Check sheet for the modelled part. Datum: model origin and axes. Units: mm. A direction names the side the tool comes from. Give positions to 0.01 mm unless a question says otherwise; leave off trailing zeros. Write each loop counter-clockwise with the first axis right and the second up, starting at its lowest first coordinate (ties: lowest second). Pieces come first, ordered by that corner, then holes. Notation, with made-up numbers: (15, 47) -> (41, 47) arc R26 cw to (41, 78) -> close; hole circle Ø9 at (36.25, 55). An arc over 180 degrees is marked (long way). Answer as a JSON object with one key per item and string values.
Autodesk Inventor part; units mm, degrees
ref_plane "Work Plane2" through (-40.9959, 0.8639, 22.2359) normal (0, 0, 1) x (1, 0, 0)
ref_plane "YZ Plane" through (0, 0, 0) normal (1, 0, 0) x (0, 1, 0)
ref_plane "XZ Plane" through (0, 0, 0) normal (0, 1, 0) x (-1, 0, 0)
ref_plane "Work Plane1" through (0, 0, 10) normal (0, 0, 1) x (1, 0, 0)
sketch "Sketch1" plane through (0, 0, 10) normal (0, 0, 1) x (1, 0, 0)
  line L0 (-4.0299, -0.3538) -> (-2.2322, 1.4439) construction
  arc A0 (-1.4439, 2.2322) -> (-2.2322, 1.4439) centre (-0.9299, 0.9299) ccw construction
  line L1 (-1.4439, 2.2322) -> (0.3538, 4.0299) construction
  line L2 (-37.8299, 42.8299) -> (-37.8299, 37.8299) construction
  line L3 (-37.8299, 37.8299) -> (-42.9208, 37.8299) construction
  line L4 (-37.8299, 42.2137) -> (-37.8299, 45.8299) construction
  line L5 (-37.8299, 45.8299) -> (-4.0299, 45.8299) construction
  line L6 (-4.0299, 45.8299) -> (-4.0299, 42.2137) construction
  line L7 (-4.0299, 4.0299) -> (0.3538, 4.0299)
  circle A1 centre (-20.9299, 20.9299) radius 17.5
  line L8 (-20.9299, 58.9723) -> (17.1124, 20.9299) construction
  line L9 (17.1124, 20.9299) -> (-20.9299, -17.1124) construction
  line L10 (-20.9299, -17.1124) -> (-58.9723, 20.9299) construction
  line L11 (-58.9723, 20.9299) -> (-20.9299, 58.9723) construction
  line L12 (-20.9299, 58.9723) -> (-20.9299, -17.1124) construction
  line L13 (17.1124, 20.9299) -> (-58.9723, 20.9299) construction
  line L14 (-20.9299, 58.9723) -> (32.8701, 58.9723) construction
  line L15 (-43.4299, 43.4299) -> (1.5701, 43.4299) construction
  line L16 (1.5701, 43.4299) -> (1.5701, -1.5701) construction
  line L17 (1.5701, -1.5701) -> (-43.4299, -1.5701) construction
  line L18 (-43.4299, -1.5701) -> (-43.4299, 43.4299) construction
  line L19 (-43.4299, 43.4299) -> (1.5701, -1.5701) construction
  line L20 (1.5701, 43.4299) -> (-43.4299, -1.5701) construction
  line L21 (-43.4299, 5.3876) -> (-43.4299, 36.4723)
  line L22 (-43.4299, 36.4723) -> (-36.4723, 43.4299)
  line L23 (-36.4723, 43.4299) -> (-5.3876, 43.4299)
  line L24 (-5.3876, 43.4299) -> (1.5701, 36.4723)
  line L25 (1.5701, 36.4723) -> (1.5701, 5.3876)
  line L26 (1.5701, 5.3876) -> (-5.3876, -1.5701)
  line L27 (-5.3876, -1.5701) -> (-36.4723, -1.5701)
  line L28 (-36.4723, -1.5701) -> (-43.4299, 5.3876)
  line L29 (-4.0299, 42.2137) -> (-37.8299, 42.2137)
  line L30 (-4.0299, -0.3538) -> (-4.0299, 4.0299)
  point P0 (-37.8299, 4.0299)
  point P1 (-20.9299, 20.9299)
  dimension "d18" = 53.8
  dimension "d19" = 45
  dimension "d20" = 53.8
  dimension "d21" = 45
  dimension "d22" = 45
extrude "Extrusion1" add sketch "Sketch1" along normal blind 5
sketch "Sketch2" plane through (0, 0, 15) normal (0, 0, 1) x (1, 0, 0)
  circle A0 centre (-35.9299, 35.9299) radius 3.0099 construction
  circle A1 centre (-5.93, 35.9299) radius 3.0099 construction
  circle A2 centre (-5.93, 5.93) radius 3.0099 construction
  circle A3 centre (-35.9299, 5.93) radius 3.0099 construction
  circle A4 centre (-35.9299, 35.9299) radius 2.7099
  circle A5 centre (-5.93, 35.9299) radius 2.7099
  circle A6 centre (-5.93, 5.93) radius 2.7099
  circle A7 centre (-35.9299, 5.93) radius 2.7099
  point P0 (0, 0)
  dimension "d_1" = 0.3
  dimension "d13" = 0.3
  dimension "d14" = 0.3
  dimension "d15" = 0.3
ref_plane "Work Plane2" through (-40.9959, 0.8639, 22.2359) normal (0, 0, 1) x (1, 0, 0)
extrude "Extrusion2" add sketch "Sketch2" along normal up to surface (7.2359 mm away)
sketch "Sketch3" plane through (0, 0, 10) normal (0, 0, -1) x (-1, 0, 0)
  line L0 (37.8299, -0.4701) -> (37.8299, 4.0299) construction
  line L1 (4.0299, 4.0299) -> (4.0299, -0.4701) construction
  line L2 (37.8299, -0.4701) -> (37.8299, 1.1886) construction
  line L3 (4.0299, -3.9701) -> (4.0299, -0.3538) construction
  line L4 (45.8299, 4.0299) -> (42.2137, 4.0299) construction
  line L5 (-0.3538, 4.0299) -> (-3.9701, 4.0299) construction
  line L6 (-3.9701, 37.8299) -> (-0.3538, 37.8299) construction
  line L7 (4.0299, 42.2137) -> (4.0299, 45.8299) construction
  line L8 (37.8299, 45.8299) -> (37.8299, 42.2137) construction
  line L9 (42.2137, 37.8299) -> (45.8299, 37.8299) construction
  line L10 (37.8299, 37.7299) -> (45.8299, 37.7299)
  line L11 (45.8299, 37.7299) -> (45.8299, 4.1299)
  line L12 (45.8299, 4.1299) -> (37.8299, 4.1299)
  line L13 (37.8299, 4.1299) -> (37.8299, 37.7299)
  line L14 (37.7299, 4.0299) -> (4.1299, 4.0299)
  line L15 (4.1299, 4.0299) -> (4.1299, -3.9701)
  line L16 (4.1299, -3.9701) -> (37.7299, -3.9701)
  line L17 (37.7299, -3.9701) -> (37.7299, 4.0299)
  line L18 (4.0299, 4.1299) -> (-3.9701, 4.1299)
  line L19 (-3.9701, 4.1299) -> (-3.9701, 37.7299)
  line L20 (-3.9701, 37.7299) -> (4.0299, 37.7299)
  line L21 (4.0299, 37.7299) -> (4.0299, 4.1299)
  line L22 (4.1299, 37.8299) -> (37.7299, 37.8299)
  line L23 (37.7299, 37.8299) -> (37.7299, 45.8299)
  line L24 (37.7299, 45.8299) -> (4.1299, 45.8299)
  line L25 (4.1299, 45.8299) -> (4.1299, 37.8299)
  point P0 (0, 0)
  dimension "d23" = 0.1
  dimension "d24" = 0.1
  dimension "d25" = 0.1
  dimension "d26" = 0.1
  dimension "d27" = 0.1
extrude "Extrusion3" add sketch "Sketch3" against normal up to surface (5 mm away)
sketch "Sketch4" plane through (0, 0, 15) normal (0, 0, 1) x (1, 0, 0)
  arc A0 (-16.3868, 4.0299) -> (-4.0299, 16.3868) centre (-20.9299, 20.9299) ccw
  line L0 (-25.4731, 4.0299) -> (-16.3868, 4.0299)
  arc A1 (-37.8299, 16.3868) -> (-25.4731, 4.0299) centre (-20.9299, 20.9299) ccw
  line L1 (-37.8299, 25.4731) -> (-37.8299, 16.3868)
  arc A2 (-25.4731, 37.8299) -> (-37.8299, 25.4731) centre (-20.9299, 20.9299) ccw
  line L2 (-16.3868, 37.8299) -> (-25.4731, 37.8299)
  arc A3 (-4.0299, 25.4731) -> (-16.3868, 37.8299) centre (-20.9299, 20.9299) ccw
  line L3 (-4.0299, 16.3868) -> (-4.0299, 25.4731)
  circle A4 centre (-5.93, 5.93) radius 2.7099
  circle A5 centre (-5.93, 35.9299) radius 2.7099
  circle A6 centre (-35.9299, 35.9299) radius 2.7099
  circle A7 centre (-35.9299, 5.93) radius 2.7099
  line L4 (3.9701, 4.1299) -> (0.3124, 4.1299)
  line L5 (3.9701, 37.7299) -> (3.9701, 4.1299)
  line L6 (0.3124, 37.7299) -> (3.9701, 37.7299)
  line L7 (0.3124, 37.7299) -> (-4.1299, 42.1723)
  line L8 (-4.1299, 45.8299) -> (-4.1299, 42.1723)
  line L9 (-37.7299, 45.8299) -> (-4.1299, 45.8299)
  line L10 (-37.7299, 42.1723) -> (-37.7299, 45.8299)
  line L11 (-37.7299, 42.1723) -> (-42.1723, 37.7299)
  line L12 (-45.8299, 37.7299) -> (-42.1723, 37.7299)
  line L13 (-45.8299, 4.1299) -> (-45.8299, 37.7299)
  line L14 (-42.1723, 4.1299) -> (-45.8299, 4.1299)
  line L15 (-42.1723, 4.1299) -> (-37.7299, -0.3124)
  line L16 (-37.7299, -3.9701) -> (-37.7299, -0.3124)
  line L17 (-4.1299, -3.9701) -> (-37.7299, -3.9701)
  line L18 (-4.1299, -0.3124) -> (-4.1299, -3.9701)
  line L19 (-4.1299, -0.3124) -> (0.3124, 4.1299)
  line L20 (-4.0299, 45.9299) -> (-4.0299, 42.2137)
  line L21 (-4.0299, 42.2137) -> (0.3538, 37.8299)
  line L22 (0.3538, 37.8299) -> (4.0701, 37.8299)
  line L23 (4.0701, 37.8299) -> (4.0701, 4.0299)
  line L24 (4.0701, 4.0299) -> (0.3538, 4.0299)
  line L25 (0.3538, 4.0299) -> (-4.0299, -0.3538)
  line L26 (-4.0299, -0.3538) -> (-4.0299, -4.0701)
  line L27 (-4.0299, -4.0701) -> (-37.8299, -4.0701)
  line L28 (-37.8299, -4.0701) -> (-37.8299, -0.3538)
  line L29 (-37.8299, -0.3538) -> (-42.2137, 4.0299)
  line L30 (-42.2137, 4.0299) -> (-45.9299, 4.0299)
  line L31 (-45.9299, 4.0299) -> (-45.9299, 37.8299)
  line L32 (-45.9299, 37.8299) -> (-42.2137, 37.8299)
  line L33 (-42.2137, 37.8299) -> (-37.8299, 42.2137)
  line L34 (-37.8299, 42.2137) -> (-37.8299, 45.9299)
  line L35 (-37.8299, 45.9299) -> (-4.0299, 45.9299)
  point P0 (0, 0)
  dimension "d18" = 53.8
  dimension "d19" = 45
  dimension "d20" = 53.8
  dimension "d21" = 45
  dimension "d22" = 45
  dimension "d30" = 0.1
extrude "Extrusion4" add sketch "Sketch4" against normal up to surface (5 mm away) contours L20 L21 L22 L23 L24 L25 L26 L27 L28 L29 L30 L31 L32 L33 L34 L35
equation "\"d13\" = d_1"
equation "\"d14\" = d_1"
equation "\"d15\" = d_1"
properties part number "50_Cube_Insert_Thorlabs"
1. Sectioned sample at C-C, the plane y = 12.5. Enter the section's corners in (x, z).
Determined:
{"outline": "(-45.93, 10) -> (-36.27, 10) -> (-36.27, 15) -> (-45.93, 15) -> close; (-5.59, 10) -> (4.07, 10) -> (4.07, 15) -> (-5.59, 15) -> close"}
2. Scan lines: L1, parallel to X at y = 36, z = 15.5; L2, parallel to Y at x = -36, z = 18; L3, parallel to Z at x = 0.5, y = 20. Record each from-to range of solid material in increasing order. Write a range as [from, to].
Determined:
{"L1": "[-38.64, -33.22], [-8.64, -3.22]", "L2": "[3.22, 8.64], [33.22, 38.64]", "L3": "[10, 15]"}
3. Sectioned sample at B-B, the plane z = 13.5. Enter the section's corners in (x, y), plus the area to 3 significant figures.
Determined:
{"outline": "(-45.93, 4.03) -> (-42.21, 4.03) -> (-37.83, -0.35) -> (-37.83, -4.07) -> (-4.03, -4.07) -> (-4.03, -0.35) -> (0.35, 4.03) -> (4.07, 4.03) -> (4.07, 37.83) -> (0.35, 37.83) -> (-4.03, 42.21) -> (-4.03, 45.93) -> (-37.83, 45.93) -> (-37.83, 42.21) -> (-42.21, 37.83) -> (-45.93, 37.83) -> close; hole (-37.83, 16.39) arc R17.5 ccw to (-25.47, 4.03) -> (-16.39, 4.03) arc R17.5 ccw to (-4.03, 16.39) -> (-4.03, 25.47) arc R17.5 ccw to (-16.39, 37.83) -> (-25.47, 37.83) arc R17.5 ccw to (-37.83, 25.47) -> close", "area": "1,330 mm^2"}
4. Mould release check, pull along X, two halves, no side actions. Record for faces 4 (the face through (-37.83, 21, 12)), 5 (the face through (-37.83, 44, 13)), 6 (the face through (-4.03, 44, 13)): released by +X, released by -X, zero draft, split by the parting line, or undercut.
Determined:
{"face 4": "undercut", "face 5": "released by -X", "face 6": "released by +X"}
5. Sectioned sample at D-D, the plane y = 5.93. Enter the section's corners in (x, z), plus the area to 3 significant figures.
Determined:
{"outline": "(-45.93, 10) -> (-29.94, 10) -> (-29.94, 15) -> (-33.22, 15) -> (-33.22, 22.24) -> (-38.64, 22.24) -> (-38.64, 15) -> (-45.93, 15) -> close; (-11.92, 10) -> (4.07, 10) -> (4.07, 15) -> (-3.22, 15) -> (-3.22, 22.24) -> (-8.64, 22.24) -> (-8.64, 15) -> (-11.92, 15) -> close", "area": "238 mm^2"}
6. Sectioned sample at A-A, the plane x = -20. Enter the section's corners in (y, z).
Determined:
{"outline": "(-4.07, 10) -> (4.03, 10) -> (4.03, 15) -> (-4.07, 15) -> close; (37.83, 10) -> (45.93, 10) -> (45.93, 15) -> (37.83, 15) -> close"}
7. Access from +Z, -Z, +X, -X, +Y, -Y to the whole of each face (thin tool, end or side, straight path). Record for faces 1 (the face through (-8.465, 8.646, 12.465)), 2 (the face through (-38, 21, 15)), 3 (the face through (-4.03, -2, 13)).
Determined:
{"face 1": "+Z, -Z", "face 2": "+Z", "face 3": "+Z, -Z, +X, -Y"}
8. Go/stop test with flat-tipped pins: P1, Ø4, axis at y = -3, z = 11.5, coming from the +X side; P2, Ø2, axis at x = -36.5, z = 16.5, coming from the -Y side; P3, Ø1.1, axis at x = -43, z = 12, coming from the -Y side. Record where each tip stops, or that it passes through.
Determined:
{"P1": "x = -4.03", "P2": "y = 3.22", "P3": "y = 4.03"}
